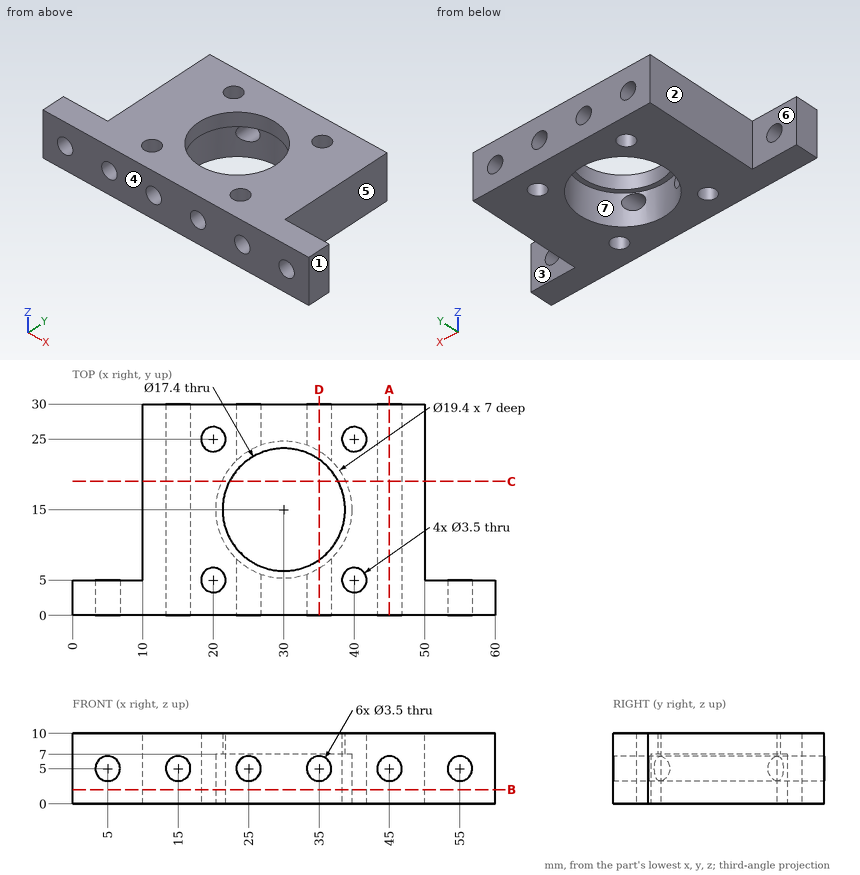
Study the drawing (mm; zero at the part's minimum x, y, z) and answer. A direction names the side the tool comes from. Round coordinates to 2 decimals unless told otherwise and drop trailing zeros. Order: outer loops, then holes, each group sorted by start corner. A loop starts at its lowest first (then second) coordinate and runs counter-clockwise, first axis right, second up. Notation, with made-up numbers: (-23.75, 28.5) -> (-7.75, 28.5) arc R26 ccw to (-7.75, 47.5) -> close; hole circle Ø10 at (11.25, -16). An arc over 180 degrees is marked (long way). Answer as CSV lines item,"result". Start each with the question number.
(1) Find the intervals of material crossed by probe 1 along Y at (x, z) = (20, 6.5); probe 2 along Z at (x, y) = (25, 27.5); probe 3 along X at (y, z) = (13.5, 5), in increasing order. Write a range as from..to.
(2) Flat-ended cylindrical pins translate along their axes: pin 1 Ø6 at (x, z) = (9.5, 9) entering from +Y; pin 2 Ø1.5 at (y, z) = (19.5, 7.5) entering from +X; pin 3 Ø3 at (x, z) = (5, 4) entering from +Y; pin 4 Ø3 at (y, z) = (19, 3.5) entering from -X. Find the tip coordinate at first contact, or state that the pin passes through.
(3) The part is cut by section D-D (x = 35). Determine the outline of the cut face in (y, z), then the cut area to 3 significant figures.
(4) A tool of negligible diameter and unlimited length cuts with its end or side. For the marked faces 1, 2 and 3, from which of +Z, -Z, +X, -X, +Y, -Y can it reach the whole face along a straight path? Write none if from no direction.
(5) For a pull along Y with two mould halves and no side action, classify the marked faces 4, 5, 6 and 7 as +Y half, -Y half, draft (parallel to the pull), parting line (faces both ways), or undercut.
(6) The part is cut by section C-C (y = 19). Determine the outline of the cut face in (x, z).
(7) The part is cut by section A-A (x = 45). Determine the outline of the cut face in (y, z), then the cut area to 3 significant figures.
(8) The part is cut by section B-B (z = 2). Determine the outline of the cut face in (x, y), then the cut area to 3 significant figures.
Evaluation:
1,probe 1,"0..3.25, 6.75..23.25, 26.75..30"
1,probe 2,"0..3.25, 6.75..10"
1,probe 3,"10..13.25, 16.75..20.42, 39.58..43.25, 46.75..50"
2,pin 1,"y = 30"
2,pin 2,"x = 50"
2,pin 3,"y = 5"
2,pin 4,"x = 10"
3,outline,"(0, 0) -> (6.69, 0) -> (6.69, 3.25) -> (0, 3.25) -> close; (0, 6.75) -> (6.69, 6.75) -> (6.69, 7) -> (7.88, 7) -> (7.88, 10) -> (0, 10) -> close; (22.12, 7) -> (23.31, 7) -> (23.31, 6.75) -> (30, 6.75) -> (30, 10) -> (22.12, 10) -> close; (23.31, 0) -> (30, 0) -> (30, 3.25) -> (23.31, 3.25) -> close"
3,area,"94.1 mm²"
4,face 1,"+Z, -Z, +X, +Y, -Y"
4,face 2,"+Z, -Z, -X, +Y"
4,face 3,"+Z, -Z, +X, +Y"
5,face 4,"-Y half"
5,face 5,"draft"
5,face 6,"+Y half"
5,face 7,"undercut"
6,outline,"(10, 0) -> (21.16, 0) -> (21.16, 7) -> (22.27, 7) -> (22.27, 10) -> (10, 10) -> close; (37.73, 7) -> (38.84, 7) -> (38.84, 0) -> (50, 0) -> (50, 10) -> (37.73, 10) -> close; hole circle Ø3.5 at (15, 5); hole circle Ø3.5 at (45, 5)"
7,outline,"(0, 0) -> (30, 0) -> (30, 3.25) -> (0, 3.25) -> close; (0, 6.75) -> (30, 6.75) -> (30, 10) -> (0, 10) -> close"
7,area,"195 mm²"
8,outline,"(0, 0) -> (60, 0) -> (60, 5) -> (50, 5) -> (50, 30) -> (10, 30) -> (10, 5) -> (0, 5) -> close; hole circle Ø3.5 at (20, 5); hole circle Ø3.5 at (20, 25); hole circle Ø19.4 at (30, 15); hole circle Ø3.5 at (40, 5); hole circle Ø3.5 at (40, 25)"
8,area,"966 mm²"
